```python
from build123d import *

# Parameters (mm, degrees)
F1_DEPTH       = 25.4
F3_D           = 4.2
F3_DEPTH       = 3.8
F3_TIP         = 1.2618073
F5_D           = 5.1054
F5_CSINK_D     = 10.4394
F5_CSINK_ANGLE = 82
F6_D           = 5.1054
F6_CSINK_D     = 10.4394
F6_CSINK_ANGLE = 82


with BuildPart() as f1:
    # F0 (on Top) → F1 (new body)
    with BuildSketch(Plane.XY):
        Polygon((15.702072531, 8.0274641514), (0, 8.0274641514), (-15.702072531, 8.0274641514), (-12.3291922584, 2.1854641514), (0, 2.1854641514), (12.3291922584, 2.1854641514), align=None)
        Polygon((0, 2.1854641514), (-12.3291922584, 2.1854641514), (-30.4818786681, 2.1854641514), (-30.4818786681, -4.6725358486), (30.5205043405, -4.6725358486), (30.5205043405, 2.1854641514), (30.4818786681, 2.1854641514), (12.3291922584, 2.1854641514), align=None)
    extrude(amount=F1_DEPTH)

    # F3
    with Locations(Plane(origin=(0, 0, 0), x_dir=(1, 0, 0), z_dir=(0, 0, -1))):
        with Locations((0, -4.0274641514)):
            Hole(F3_D / 2, depth=F3_DEPTH)
            with Locations((0, 0, -(F3_DEPTH + F3_TIP / 2))):  # 118° drill point
                Cone(0, F3_D / 2, F3_TIP, mode=Mode.SUBTRACT)

    # F5 (through all)
    with Locations(Plane(origin=(0, 8.0274641514, 0), x_dir=(-1, 0, 0), z_dir=(0, 1, 0))):
        with Locations((0, 19.812)):
            CounterSinkHole(F5_D / 2, F5_CSINK_D / 2, counter_sink_angle=F5_CSINK_ANGLE)

    # F6 (through all)
    with Locations(Plane(origin=(0, 8.0274641514, 0), x_dir=(-1, 0, 0), z_dir=(0, 1, 0))):
        with Locations((0, 8.636)):
            CounterSinkHole(F6_D / 2, F6_CSINK_D / 2, counter_sink_angle=F6_CSINK_ANGLE)


solid = f1.part
```
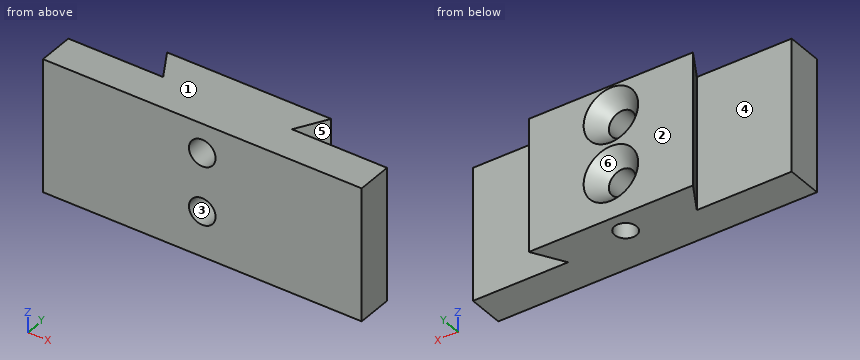
Verification items for the finished model (mm, model axes). Face numbers are marked on the shaded views. A direction names the side the tool comes from. Coordinates: 2 decimals unless noted, no trailing zeros. Loops run counter-clockwise (first coordinate to the right, second up) from the corner with the lowest first, then second, coordinate; pieces in that order, holes last. Notation, with made-up numbers: (24.5, 44) -> (61.5, 44) arc R17 cw to (61.5, 48) -> close; hole circle Ø9 at (7.5, 35). An arc over 180 degrees is marked (long way). Put each result on its own line as item: value.
1. Section check B-B, the plane x = -1.5. Give the number of separate pieces and of enclosed holes in the cut face, then the cut area to 3 significant figures.
Result set:
separate pieces: 3
enclosed holes: 0
area: 187 mm^2
2. Thickness scan on line 1 (Y direction, x = 0, z = 2.3); line 2 (Z direction, x = 0, y = 2.5); line 3 (Z direction, x = 0, y = 2). Record the ranges inside material, lowest first.
Result set:
line 1: y = -4.67 to 1.93, 6.13 to 8.03
line 2: z = 4.14 to 6.08, 11.19 to 17.26, 22.36 to 25.4
line 3: z = 3.84 to 6.08, 11.19 to 17.26, 22.36 to 25.4
3. Section check A-A, the plane x = -20.5. Record the boundary of the cut face in (y, z), then the cut area to 3 significant figures.
Result set:
outline: (-4.67, 0) -> (2.19, 0) -> (2.19, 25.4) -> (-4.67, 25.4) -> close
area: 174 mm^2
4. Mould release check, pull along Z, two halves, no side actions. Record for the marked faces 1, 2 and 3: pulls with the +Z half, pulls with the -Z half, needs draft (parallel to the pull), parting line crosses it, or undercut.
Result set:
face 1: pulls with the +Z half
face 2: needs draft
face 3: undercut
5. Tool access check on the marked faces 4, 5 and 6. Record the directions out of +Z, -Z, +X, -X, +Y, -Y that give a thin tool (end or side, any length) a straight path to the whole face; none if there is none.
Result set:
face 4: +Z, -Z, -X
face 5: +Z, -Z, +X
face 6: +Y
6. Gauge pin test, flat ends, axial feed: P1, Ø4.5, axis at x = 0, z = 19.812, coming from the -Y side; P2, Ø3, axis at y = 6.5, z = 8, coming from the -X side; P3, Ø4, axis at x = 0, y = 4.03, coming from the -Z side. Record the tip position at first contact, or that the pin passes through.
Result set:
P1: passes through
P2: stops at x = -15.69
P3: stops at z = 3.86
